Source: CAD feature listing. Evaluate the final solid. Frame: model axes, mm. A direction names the side the tool comes from. Round coordinates to 2 decimals unless told otherwise and drop trailing zeros. Order: outer loops, then holes, each group sorted by start corner. A loop starts at its lowest first (then second) coordinate and runs counter-clockwise, first axis right, second up. Notation, with made-up numbers: (40.25, 87.25) -> (59.25, 87.25) arc R19 cw to (59.25, 100.25) -> close; hole circle Ø2 at (43, 60.5). An arc over 180 degrees is marked (long way). One line per item, written item: value. Start each with the question number.
1) Section A-A (y = 4.75). State how many separate pieces and enclosed holes the cut face has, and give its area (3 significant figures).
2) Section C-C (y = 2). Return the cut outline in (x, z).
3) Section D-D (z = -5). Return the cut outline in (x, y), and give its area (3 significant figures).
4) Pin query (flat end, axial travel): P1, Ø3, axis at x = -3.3, y = 6, coming from the +Z side; P2, Ø4.5, axis at x = 24.5, y = 9, coming from the -Z side; P3, Ø10, axis at x = 3, z = -22, coming from the -Y side; P4, Ø0.6, axis at x = -2, z = -3.5, coming from the +Y side. Return the tip coordinate at first contact, or that it passes through.
5) Ray query, L1, parallel to Y at x = 26.3, z = -17.1; L2, parallel to Z at x = 16, y = 6.75; L3, parallel to Z at x = 3, y = 2.5. Return the intervals inside material, ascending.
6) Mould query, pull axis X, two halves, no side actions, for faces 1 (the face through (7.474, 7.352, -27.479)), 2 (the face through (-1, 6, -18)), 3 (the face through (24.55, 5.93, -17.01)), 4 (the face through (19.507, 5.916, -20.028)). Classes: pulls with the +X half, pulls with the -X half, needs draft (parallel to the pull), parting line crosses it, or undercut.
7) Reachability of faces 5 (the face through (-1, 6, -2)), 6 (the face through (0, 6, -20)), 7 (the face through (1, 1, -22)) from +Z, -Z, +X, -X, +Y, -Y: full face, straight path, thin tool, end or side. Return the list, or none.
```python
from build123d import *

# Parameters (mm, degrees)
BOSS_EXTRU_1_DEPTH      = 12
BOSS_EXTRU_2_DEPTH      = 5
BOSS_EXTRU_2_DEPTH_BACK = 28
ESQUISSE2_W             = 2
ESQUISSE2_H             = 12
ESQUISSE3_R             = 1.75
ENL_V_MAT_EXTRU_2_DEPTH = 5
ESQUISSE4_R             = 1.75
ENL_V_MAT_EXTRU_3_DEPTH = 5
ESQUISSE5_R             = 6
BOSS_EXTRU_3_DEPTH      = 4
ESQUISSE6_R             = 2
BOSS_EXTRU_4_DEPTH      = 3
ESQUISSE7_W             = 2
ESQUISSE7_H             = 5
BOSS_EXTRU_5_DEPTH      = 3


with BuildPart() as part:
    # Esquisse1 → Boss.-Extru.1 (new body)
    with BuildSketch(Plane(origin=(0, 0, 0), x_dir=(1, 0, 0), z_dir=(0, 1, 0))):
        Polygon((17, 22), (23, 17.279676248), (23, 0), (0, 0), (0, 22), align=None)
    extrude(amount=BOSS_EXTRU_1_DEPTH)

    # Esquisse2 → Boss.-Extru.2 (add, two sides: drawn at the far end of the back side and taken through both)
    with BuildSketch(Plane.ZY.offset(-BOSS_EXTRU_2_DEPTH_BACK)):
        with Locations((-17, 6)):
            Rectangle(ESQUISSE2_W, ESQUISSE2_H)
    extrude(amount=BOSS_EXTRU_2_DEPTH + BOSS_EXTRU_2_DEPTH_BACK)

    # Esquisse3 → Enlèv. mat.-Extru.2 (cut)
    with BuildSketch(Plane(origin=(0, 0, -18), x_dir=(-1, 0, 0), z_dir=(0, 0, -1))):
        with Locations((3.3, 6)):
            Circle(ESQUISSE3_R)
    extrude(amount=-ENL_V_MAT_EXTRU_2_DEPTH, mode=Mode.SUBTRACT)

    # Esquisse4 → Enlèv. mat.-Extru.3 (cut)
    with BuildSketch(Plane(origin=(0, 0, -18), x_dir=(-1, 0, 0), z_dir=(0, 0, -1))):
        with Locations((-26.3, 6)):
            Circle(ESQUISSE4_R)
    extrude(amount=-ENL_V_MAT_EXTRU_3_DEPTH, mode=Mode.SUBTRACT)

    # Esquisse5 → Boss.-Extru.3 (add)
    with BuildSketch(Plane(origin=(0, 0, -22), x_dir=(-1, 0, 0), z_dir=(0, 0, -1))):
        with Locations((-6, 6)):
            Circle(ESQUISSE5_R)
    extrude(amount=BOSS_EXTRU_3_DEPTH)

    # Esquisse6 → Boss.-Extru.4 (add)
    with BuildSketch(Plane(origin=(0, 0, -26), x_dir=(-1, 0, 0), z_dir=(0, 0, -1))):
        with Locations((-6, 6)):
            Circle(ESQUISSE6_R)
    extrude(amount=BOSS_EXTRU_4_DEPTH)

    # Esquisse7 → Boss.-Extru.5 (add)
    with BuildSketch(Plane.ZY):
        with Locations((-3, 6)):
            Rectangle(ESQUISSE7_W, ESQUISSE7_H)
    extrude(amount=BOSS_EXTRU_5_DEPTH)


solid = part.part
```
Findings:
1. separate pieces: 3
1. enclosed holes: 0
1. area: 565 mm2
2. outline: (-5, -18) -> (0, -18) -> (0, -22) -> (1.53, -22) -> (1.53, -26) -> (10.47, -26) -> (10.47, -22) -> (17, -22) -> (22.08, -18) -> (28, -18) -> (28, -16) -> (23, -16) -> (23, 0) -> (0, 0) -> (0, -16) -> (-5, -16) -> close
3. outline: (0, 0) -> (23, 0) -> (23, 12) -> (0, 12) -> close
3. area: 276 mm2
4. P1: z = -2
4. P2: z = -18
4. P3: y = 0
4. P4: y = 8.5
5. L1: 0 to 4.25, 7.75 to 12
5. L2: -22 to 0
5. L3: -26 to 0
6. face 1: parting line crosses it
6. face 2: needs draft
6. face 3: undercut
6. face 4: pulls with the +X half
7. face 5: +Z, -X, +Y, -Y
7. face 6: -Z, -X, +Y, -Y
7. face 7: -Z, -X, -Y
